Design review of the part built by this model. Coordinates are the model's own, in mm. A direction names the side the tool comes from. Give positions to 0.01 mm unless a question says otherwise; leave off trailing zeros. Write each loop counter-clockwise with the first axis right and the second up, starting at its lowest first coordinate (ties: lowest second). Pieces come first, ordered by that corner, then holes. Notation, with made-up numbers: M 12,-40 L 66,-40 A32 cw 66,-3 Z; hole C -14.75,80.5 d4. An arc over 180 degrees is marked long. Answer in a Markdown table with one row per item.
```python
from build123d import *

# Parameters (mm, degrees)
SKETCH1_R           = 381
SKETCH1_R_2         = 374.65
BOSS_EXTRUDE1_DEPTH = 1066.8
SKETCH4_W           = 127
SKETCH4_H           = 203.2
SKETCH4_W_2         = 203.2
SKETCH4_H_2         = 127
CUT_EXTRUDE7_DEPTH  = 127
SKETCH6_W           = 203.2
SKETCH6_H           = 127
SKETCH6_W_2         = 183.106953235
SKETCH6_H_2         = 114.441845772
SKETCH6_W_3         = 127
SKETCH6_H_3         = 203.2
SKETCH6_W_4         = 114.441845772
SKETCH6_H_4         = 183.106953235
BOSS_EXTRUDE3_DEPTH = 127
SKETCH7_W           = 199.503476618
SKETCH7_H           = 127
SKETCH7_W_2         = 127
SKETCH7_H_2         = 199.503476618
BOSS_EXTRUDE4_DEPTH = 6.35
SKETCH8_R           = 381
BOSS_EXTRUDE5_DEPTH = 6.35


with BuildPart() as part:
    # Sketch1 → Boss-Extrude1 (new body)
    with BuildSketch(Plane(origin=(0, 0, 0), x_dir=(1, 0, 0), z_dir=(0, 1, 0))):
        Circle(SKETCH1_R)
        Circle(SKETCH1_R_2, mode=Mode.SUBTRACT)
    extrude(amount=BOSS_EXTRUDE1_DEPTH)

    # Sketch3 → Revolve1 (revolve)
    with BuildSketch(Plane.XY):
        Polygon((203.2, 1066.8), (381, 939.8), (381, 931.996462079), (201.165046911, 1060.45), (101.6, 1060.45), (101.6, 1066.8), align=None)
    revolve(axis=Axis((0, 1066.8, 0), (0, -1, 0)))

    # Sketch5 → Cut-Revolve2 (revolve, cut)
    with BuildSketch(Plane.XY):
        Polygon((203.2, 1066.8), (381, 939.8), (381, 1066.8), align=None)
    revolve(axis=Axis((0, 0, 0), (0, 1, 0)), mode=Mode.SUBTRACT)

    # Sketch4 → Cut-Extrude7 (cut)
    with BuildSketch(Plane(origin=(0, 1066.8, 0), x_dir=(1, 0, 0), z_dir=(0, 1, 0))):
        with Locations((0, -274.071066227)):
            Rectangle(SKETCH4_W, SKETCH4_H)
        with Locations((274.071066227, 0)):
            Rectangle(SKETCH4_W_2, SKETCH4_H_2)
        with Locations((-274.071066227, 0)):
            Rectangle(SKETCH4_W_2, SKETCH4_H_2)
        with Locations((0, 274.071066227)):
            Rectangle(SKETCH4_W, SKETCH4_H)
    extrude(amount=-CUT_EXTRUDE7_DEPTH, mode=Mode.SUBTRACT)

    # Sketch6 → Boss-Extrude3 (add)
    with BuildSketch(Plane(origin=(0, 1066.8, 0), x_dir=(1, 0, 0), z_dir=(0, 1, 0))):
        with Locations((274.071066227, 0)):
            Rectangle(SKETCH6_W, SKETCH6_H)
        with Locations((274.071066227, 0)):
            Rectangle(SKETCH6_W_2, SKETCH6_H_2, mode=Mode.SUBTRACT)
        with Locations((0, -274.071066227)):
            Rectangle(SKETCH6_W_3, SKETCH6_H_3)
        with Locations((0, -274.071066227)):
            Rectangle(SKETCH6_W_4, SKETCH6_H_4, mode=Mode.SUBTRACT)
        with Locations((-274.071066227, 0)):
            Rectangle(SKETCH6_W, SKETCH6_H)
        with Locations((-274.071066227, 0)):
            Rectangle(SKETCH6_W_2, SKETCH6_H_2, mode=Mode.SUBTRACT)
        with Locations((0, 274.071066227)):
            Rectangle(SKETCH6_W_3, SKETCH6_H_3)
        with Locations((0, 274.071066227)):
            Rectangle(SKETCH6_W_4, SKETCH6_H_4, mode=Mode.SUBTRACT)
    extrude(amount=-BOSS_EXTRUDE3_DEPTH)

    # Sketch7 → Boss-Extrude4 (add)
    with BuildSketch(Plane(origin=(0, 1066.8, 0), x_dir=(1, 0, 0), z_dir=(0, 1, 0))):
        with Locations((275.919327918, 0)):
            Rectangle(SKETCH7_W, SKETCH7_H)
        with Locations((0, -275.919327918)):
            Rectangle(SKETCH7_W_2, SKETCH7_H_2)
        with Locations((-275.919327918, 0)):
            Rectangle(SKETCH7_W, SKETCH7_H)
        with Locations((0, 275.919327918)):
            Rectangle(SKETCH7_W_2, SKETCH7_H_2)
    extrude(amount=BOSS_EXTRUDE4_DEPTH)

    # Sketch8 → Boss-Extrude5 (add)
    with BuildSketch(Plane.XZ):
        Circle(SKETCH8_R)
    extrude(amount=BOSS_EXTRUDE5_DEPTH)

    # Sketch9 → Cut-Revolve3 (revolve, cut)
    with BuildSketch(Plane.XY):
        Polygon((172.471066227, 1060.45), (374.65, 936.532176365), (172.471066227, 936.532176365), align=None)
    revolve(axis=Axis((0, 0, 0), (0, 1, 0)), mode=Mode.SUBTRACT)


solid = part.part
```
1) For faces 4 (the face through (-277, 1073.15, -1)), 5 (the face through (23.655, 1053.466, 182.338)), 6 (the face through (-63.5, 1035, 322)), 7 (the face through (-63.5, 1035, -319)), list the 3-axis set-ups (+Z, -Z, +X, -X, +Y, -Y) from which the entire face can be reached by the end or side of a thin tool; tool diameter is ignored.
Geometry says:
| item | result |
|---|---|
| face 4 | +Z, -Z, +X, -X, +Y |
| face 5 | none |
| face 6 | +Z, -X, +Y |
| face 7 | -Z, -X, +Y |
2) Insertion check: P1, Ø1.5, axis at x = 62.5, z = 67.5, coming from the +Y side; P2, Ø8, axis at y = 916.5, z = -3.5, coming from the -X side; P3, Ø2, axis at y = 882, z = 63.5, coming from the +X side; P4, Ø4, axis at y = 503, z = 21.5, coming from the +X side. Each pin has a flat end and moves straight along its axis. Give the tip position at first contact, or say it passes through.
Geometry says:
| item | result |
|---|---|
| P1 | y = 0 |
| P2 | x = -381 |
| P3 | x = 375.84 |
| P4 | x = 380.5 |
3) Add section A-A (y = 475). Write out the cut boundary in (x, z).
Geometry says:
| item | result |
|---|---|
| outline | C 0,0 d762; hole C 0,0 d749.3 |
4) The part is to be moulded in two halves that separate along X. For faces 1 (the face through (209.213, 1002.411, 205.624)), 2 (the face through (-365.625, 1004, 1)), 3 (the face through (-1, 1006, 375.671)), say which applies: released by +X, released by -X, zero draft, split by the parting line, or undercut.
Geometry says:
| item | result |
|---|---|
| face 1 | released by +X |
| face 2 | undercut |
| face 3 | zero draft |
5) To check wall thickness, follow probe 1 along Z at (x, y) = (0, 1063); probe 2 along Y at (x, z) = (-306.5, 5); probe 3 along Z at (x, y) = (0, 449). State the ranges of each line that lie inside material, in increasing order. Write a range as [from, to].
Geometry says:
| item | result |
|---|---|
| probe 1 | [-375.67, -365.62], [-182.52, -101.6], [101.6, 182.52], [365.62, 375.67] |
| probe 2 | [-6.35, 0], [1066.8, 1073.15] |
| probe 3 | [-381, -374.65], [374.65, 381] |
